```python
from build123d import *

# Parameters (mm, degrees)
SKETCH1_R           = 11.85
BOSS_EXTRUDE1_DEPTH = 1
SKETCH2_R           = 11.85
SKETCH2_R_2         = 10.85
BOSS_EXTRUDE2_DEPTH = 9
FILLET1_R           = 0.5


with BuildPart() as part:
    # Sketch1 → Boss-Extrude1 (new body)
    with BuildSketch(Plane(origin=(0, 0, 0), x_dir=(1, 0, 0), z_dir=(0, 1, 0))):
        Circle(SKETCH1_R)
    extrude(amount=BOSS_EXTRUDE1_DEPTH)

    # Sketch2 → Boss-Extrude2 (add)
    with BuildSketch(Plane(origin=(0, 1, 0), x_dir=(1, 0, 0), z_dir=(0, 1, 0))):
        Circle(SKETCH2_R)
        Circle(SKETCH2_R_2, mode=Mode.SUBTRACT)
    extrude(amount=BOSS_EXTRUDE2_DEPTH)

    # Fillet1
    fillet1_edges = [part.edges().sort_by_distance(p)[0] for p in [
        (-11.85, 0, 0),
    ]]
    fillet(fillet1_edges, radius=FILLET1_R)


solid = part.part
```
Source: CAD feature listing. Evaluate the final solid. Frame: model axes, mm. Round coordinates to 2 decimals unless told otherwise and drop trailing zeros. Loops run counter-clockwise (first coordinate to the right, second up) from the corner with the lowest first, then second, coordinate; pieces in that order, holes last. Notation, with made-up numbers: M 26.5,39.5 L 70.5,39.5 A20 cw 70.5,68.5 Z; hole C -3,0 d6. An arc over 180 degrees is marked long. Use a Markdown table: item, result. Add a question column.
1. Cut plane A-A, the plane x = 0. Output: boundary loops of the cut face in (y, z), and give its area (3 significant figures).
2. Ray query, line 1 along X through (y, z) = (5.75, 0); line 2 along Y through (x, z) = (0.25, 7). Return the intervals inside material, ascending. Write a range as [from, to].
3. Contact query for flat-ended pins moving along their axis: pin 1 (4 mm diameter, centred on x = -9.5, y = 7, fed in from -Z); pin 2 (2 mm diameter, centred on y = 1, z = -4, fed in from +X); pin 3 (1.5 mm diameter, centred on x = -5.5, y = 6, fed in from -Z). Output: stop coordinate, or through.
4. Cut plane C-C, the plane y = 8.25. Output: boundary loops of the cut face in (x, z), and give its area (3 significant figures).
5. Pull-direction query (X, two-part tool) for faces 1 (the cylindrical face through (-8, 5.44, -7.33)), 2 (the flat face through (0, 1, 0)), 3 (the cylindrical face through (11.303, 5.184, -3.559)), 4 (the flat face through (5, 10, 10)); classes: +X half, -X half, draft (parallel to the pull), parting line (faces both ways), or undercut.
6. Cut plane B-B, the plane z = 0. Output: boundary loops of the cut face in (x, y), and give its area (3 significant figures).
Solution:
| question | item | result |
|---|---|---|
| 1 | outline | M 0,-11.35 A0.5 ccw 0.5,-11.85 L 10,-11.85 L 10,-10.85 L 1,-10.85 L 1,10.85 L 10,10.85 L 10,11.85 L 0.5,11.85 A0.5 ccw 0,11.35 Z |
| 1 | area | 41.6 mm2 |
| 2 | line 1 | x = [-11.85, -10.85], [10.85, 11.85] |
| 2 | line 2 | y = [0, 1] |
| 3 | pin 1 | stops at z = -9.17 |
| 3 | pin 2 | stops at x = 11.46 |
| 3 | pin 3 | stops at z = -10.86 |
| 4 | outline | C 0,0 d23.7; hole C 0,0 d21.7 |
| 4 | area | 71.3 mm2 |
| 5 | face 1 | undercut |
| 5 | face 2 | undercut |
| 5 | face 3 | parting line |
| 5 | face 4 | draft |
| 6 | outline | M -11.85,0.5 A0.5 ccw -11.35,0 L 11.35,0 A0.5 ccw 11.85,0.5 L 11.85,10 L 10.85,10 L 10.85,1 L -10.85,1 L -10.85,10 L -11.85,10 Z |
| 6 | area | 41.6 mm2 |
